```python
from build123d import *

# Parameters (mm, degrees)
SKETCH1_W               = 304.8
SKETCH1_H               = 304.8
BOSS_EXTRUDE1_DEPTH     = 3.175
SKETCH3_R               = 2.600000007
CUT_EXTRUDE1_DEPTH      = 4.175
SKETCH5_R               = 1.5
SKETCH5_R_2             = 2.999999969
CUT_EXTRUDE2_DEPTH      = 4.175
SKETCH7_R               = 0.999998
CUT_EXTRUDE3_DEPTH      = 4.175
SKETCH9_R               = 1.726999975
SKETCH9_R_2             = 6.35
CUT_EXTRUDE5_DEPTH      = 1
CUT_EXTRUDE5_DEPTH_BACK = 4.175
SKETCH11_R              = 1.5
SKETCH11_R_2            = 6.985
CUT_EXTRUDE6_DEPTH      = 1
CUT_EXTRUDE6_DEPTH_BACK = 4.175


with BuildPart() as part:
    # Sketch1 → Boss-Extrude1 (new body)
    with BuildSketch(Plane(origin=(0, 0, 0), x_dir=(1, 0, 0), z_dir=(0, 1, 0))):
        Rectangle(SKETCH1_W, SKETCH1_H)
    extrude(amount=BOSS_EXTRUDE1_DEPTH)

    # Sketch3 → Cut-Extrude1 (cut, through all)
    with BuildSketch(Plane(origin=(0, 3.175, 0), x_dir=(1, 0, 0), z_dir=(0, 1, 0))):
        with Locations((-146.05, -31.75)):
            Circle(SKETCH3_R)
        with Locations((-95.25, -88.9)):
            Circle(SKETCH3_R)
        with Locations((-146.05, -88.9)):
            Circle(SKETCH3_R)
    cut_extrude1 = extrude(amount=-CUT_EXTRUDE1_DEPTH, mode=Mode.SUBTRACT)

    # Mirror1: Cut-Extrude1 across plane
    add(cut_extrude1.mirror(Plane.XY), mode=Mode.SUBTRACT)

    # Sketch5 → Cut-Extrude2 (cut, through all)
    with BuildSketch(Plane(origin=(0, 3.175, 0), x_dir=(1, 0, 0), z_dir=(0, 1, 0))):
        with Locations((-66.312, 15.5)):
            Circle(SKETCH5_R)
        with Locations((-66.312, -15.5)):
            Circle(SKETCH5_R)
        with Locations((-97.312, 15.5)):
            Circle(SKETCH5_R)
        with Locations((-97.312, -15.5)):
            Circle(SKETCH5_R)
        with Locations((-81.812, 0)):
            Circle(SKETCH5_R_2)
    extrude(amount=-CUT_EXTRUDE2_DEPTH, mode=Mode.SUBTRACT)

    # Sketch7 → Cut-Extrude3 (cut, through all)
    with BuildSketch(Plane(origin=(0, 3.175, 0), x_dir=(1, 0, 0), z_dir=(0, 1, 0))):
        with Locations((46.431787507, -35.001787507)):
            Circle(SKETCH7_R)
        with Locations((-23.571787507, -35.001787507)):
            Circle(SKETCH7_R)
        with Locations((-23.571787507, 35.001787507)):
            Circle(SKETCH7_R)
        with Locations((46.431787507, 35.001787507)):
            Circle(SKETCH7_R)
    extrude(amount=-CUT_EXTRUDE3_DEPTH, mode=Mode.SUBTRACT)

    # Sketch9 → Cut-Extrude5 (cut, two sides)
    with BuildSketch(Plane(origin=(0, 3.175, 0), x_dir=(1, 0, 0), z_dir=(0, 1, 0))) as cut_extrude5_sk:
        with Locations((-131.7625, -147.6375)):
            Circle(SKETCH9_R)
        with Locations((-131.7625, -131.7625)):
            Circle(SKETCH9_R)
        with Locations((-147.6375, -131.7625)):
            Circle(SKETCH9_R)
        with Locations((-147.6375, -147.6375)):
            Circle(SKETCH9_R)
        with Locations((-139.7, -139.7)):
            Circle(SKETCH9_R_2)
        with Locations((138.1125, -94.2975)):
            Circle(SKETCH9_R)
        with Locations((138.1125, -78.4225)):
            Circle(SKETCH9_R)
        with Locations((130.175, -86.36)):
            Circle(SKETCH9_R_2)
        with Locations((122.2375, -78.4225)):
            Circle(SKETCH9_R)
        with Locations((122.2375, -94.2975)):
            Circle(SKETCH9_R)
        with Locations((122.2375, 94.2975)):
            Circle(SKETCH9_R)
        with Locations((122.2375, 78.4225)):
            Circle(SKETCH9_R)
        with Locations((138.1125, 94.2975)):
            Circle(SKETCH9_R)
        with Locations((130.175, 86.36)):
            Circle(SKETCH9_R_2)
        with Locations((138.1125, 78.4225)):
            Circle(SKETCH9_R)
        with Locations((-131.7625, 131.7625)):
            Circle(SKETCH9_R)
        with Locations((-131.7625, 147.6375)):
            Circle(SKETCH9_R)
        with Locations((-147.6375, 147.6375)):
            Circle(SKETCH9_R)
        with Locations((-147.6375, 131.7625)):
            Circle(SKETCH9_R)
        with Locations((-139.7, 139.7)):
            Circle(SKETCH9_R_2)
    extrude(amount=CUT_EXTRUDE5_DEPTH, mode=Mode.SUBTRACT)
    extrude(cut_extrude5_sk.sketch, amount=-CUT_EXTRUDE5_DEPTH_BACK, mode=Mode.SUBTRACT)

    # Sketch11 → Cut-Extrude6 (cut, two sides)
    with BuildSketch(Plane(origin=(0, 3.175, 0), x_dir=(1, 0, 0), z_dir=(0, 1, 0))) as cut_extrude6_sk:
        with Locations((26.93, 15.5)):
            Circle(SKETCH11_R)
        with Locations((26.93, -15.5)):
            Circle(SKETCH11_R)
        with Locations((-4.07, -15.5)):
            Circle(SKETCH11_R)
        with Locations((-4.07, 15.5)):
            Circle(SKETCH11_R)
        with Locations((11.43, 0)):
            Circle(SKETCH11_R_2)
    extrude(amount=CUT_EXTRUDE6_DEPTH, mode=Mode.SUBTRACT)
    extrude(cut_extrude6_sk.sketch, amount=-CUT_EXTRUDE6_DEPTH_BACK, mode=Mode.SUBTRACT)


solid = part.part
```
Geometry: final body of the model. Coordinates: model frame, mm. Coordinates: 2 decimals unless noted, no trailing zeros. Order: outer loops, then holes, each group sorted by start corner. A loop starts at its lowest first (then second) coordinate and runs counter-clockwise, first axis right, second up. Notation, with made-up numbers: (-0.5, 50.5) - (24.5, 50.5) arc R11 ccw to (24.5, 60.5) - close; hole circle Ø2 at (29.25, 6.25). An arc over 180 degrees is marked (long way). Write each question's results on one line, items separated by ' | '.
1) Section B-B, the plane z = 139.7. Return loops of the section in (x, y) (3 decimals), plus the area to 3 significant figures.
Results list:
outline: (-152.4, 0) - (-146.05, 0) - (-146.05, 3.175) - (-152.4, 3.175) - close; (-133.35, 0) - (152.4, 0) - (152.4, 3.175) - (-133.35, 3.175) - close | area: 927 mm^2
2) Pull-direction query (X, two-part tool) for faces 1 (the cylindrical face through (4.45, 1.61, -0.31)), 2 (the flat face through (-2, 3.175, -2)); classes: pulls with the +X half, pulls with the -X half, needs draft (parallel to the pull), parting line crosses it, or undercut.
Results list:
face 1: undercut | face 2: needs draft
3) Pin query (flat end, axial travel): pin 1 (4 mm diameter, centred on x = -146.05, z = -88.9, fed in from +Y). Return the tip coordinate at first contact, or that it passes through.
Results list:
pin 1: through
4) Section C-C, the plane x = 132. Return loops of the section in (y, z) (3 decimals).
Results list:
outline: (0, -152.4) - (3.175, -152.4) - (3.175, -92.442) - (0, -92.442) - close; (0, -80.278) - (3.175, -80.278) - (3.175, 80.278) - (0, 80.278) - close; (0, 92.442) - (3.175, 92.442) - (3.175, 152.4) - (0, 152.4) - close
5) Line query: line 1 (Z direction, x = -97.5, y = 1.5); line 2 (X direction, y = 2.45, z = 2.5); line 3 (X direction, y = 0.7, z = 88.9). Output: solid intervals per line, ascending. Write a range as from..to.
Results list:
line 1: -152.4..-90.2, -87.6..-16.99, -14.01..14.01, 16.99..87.6, 90.2..152.4 | line 2: -152.4..-83.47, -80.15..4.91, 17.95..152.4 | line 3: -152.4..-148.65, -143.45..-97.85, -92.65..124.36, 135.99..152.4
6) Section A-A, the plane x = -139.7. Return loops of the section in (y, z) (3 decimals), plus the area to 3 significant figures.
Results list:
outline: (0, -152.4) - (3.175, -152.4) - (3.175, -146.05) - (0, -146.05) - close; (0, -133.35) - (3.175, -133.35) - (3.175, 133.35) - (0, 133.35) - close; (0, 146.05) - (3.175, 146.05) - (3.175, 152.4) - (0, 152.4) - close | area: 887 mm^2
